```python
from build123d import *

# Parameters (mm, degrees)
F1_DEPTH = 2
F3_DEPTH = 2
F5_DEPTH = 2
F6_R     = 1


with BuildPart() as f1:
    # F0 (on Top) → F1 (new body)
    with BuildSketch(Plane.XY):
        Polygon((-13.435029, 6.363961), (-2.071068, -5), (14, -5), (14, 4), (1.656854, 4), (-7.071068, 12.727922), align=None)
    extrude(amount=F1_DEPTH)

    # F2 (on face) → F3 (join)
    with BuildSketch(Plane.XY.offset(2)):
        Polygon((-12.020815, 7.778175), (-13.435029, 6.363961), (-2.071068, -5), (14, -5), (14, -3), (-1.242641, -3), align=None)
    extrude(amount=F3_DEPTH)

    # F4 (on face) → F5 (join)
    with BuildSketch(Plane.XY.offset(4)):
        Polygon((-7.071068, 12.727922), (-12.020815, 7.778175), (-13.435029, 6.363961), (-2.071068, -5), (14, -5), (14, -3), (14, 4), (1.656854, 4), align=None)
    extrude(amount=F5_DEPTH)

    # F6
    f6_edges = [f1.edges().sort_by_distance(p)[0] for p in [
        (-13.435029, 6.363961, 3),
        (-7.753048, 0.681981, 6),
        (-2.071068, -5, 3),
        (-7.753048, 0.681981, 0),
        (5.964466, -5, 6),
        (14, -5, 3),
        (5.964466, -5, 0),
        (-10.253048, 9.545942, 0),
        (14, -0.5, 0),
        (7.828427, 4, 0),
        (-2.707107, 8.363961, 0),
        (14, -0.5, 6),
        (7.828427, 4, 6),
        (-2.707107, 8.363961, 6),
        (-10.253048, 9.545942, 6),
    ]]
    fillet(f6_edges, radius=F6_R)


solid = f1.part
```
Model file for the job. Use its own axes, mm. A direction names the side the tool comes from. Coordinates: 2 decimals unless noted, no trailing zeros. Loops run counter-clockwise (first coordinate to the right, second up) from the corner with the lowest first, then second, coordinate; pieces in that order, holes last. Notation, with made-up numbers: (36, -5.5) - (40, -5.5) arc R17 ccw to (40, 21.5) - close; hole circle Ø9 at (53, -28). An arc over 180 degrees is marked (long way). Answer as a JSON object with one key per item and string values. Group by question number.
(1) Tool access for faces 1 (the face through (5.774, -4.715, 5.699)), 2 (the face through (1, 3, 4)), 3 (the face through (7.532, 3.715, 5.699)): list every direction of +Z, -Z, +X, -X, +Y, -Y with a clear straight run to the whole face (end or side of a thin tool).
(2) Flat gauge pin, fed straight in: pin 1 (1.1 mm diameter, centred on x = 8, z = 1.5, fed in from +Y). Where does the tip first touch, or does it go through?
(3) Cut at A-A (x = 11.25). Give the cut face in (y, z), then the cut area to 3 significant figures.
(4) Probe line 1 along Z through (x, y) = (2, -1.75); line 2 along Y through (x, z) = (6.75, 1.75); line 3 along Z through (x, y) = (-10, 9.5). List the from-to ranges inside material, lowest first.
(5) Two-plate mould, pull along Z, no slides. Class faces 4 (the face through (13.715, 0.056, 5.699)), 5 (the face through (-6.556, 2.314, 2.986)), 6 (the face through (7.9, 4, 4.5)): released by +Z, released by -Z, zero draft, split by the parting line, or undercut.
(6) Cut at B-B (z = 2.5). Give the cut face in (x, y), then the cut area to 3 significant figures.
Geometry says:
{
 "1": {"face 1": "+Z, +X, -X, -Y", "face 2": "+X, +Y", "face 3": "+Z, +X, +Y"},
 "2": {"pin 1": "stops at y = 4"},
 "3": {"outline": "(-5, 1) arc R1 ccw to (-4, 0) - (3, 0) arc R1 ccw to (4, 1) - (4, 2) - (-3, 2) - (-3, 4) - (4, 4) - (4, 5) arc R1 ccw to (3, 6) - (-4, 6) arc R1 ccw to (-5, 5) - close", "area": "39.1 mm^2"},
 "4": {"line 1": "z = 0 to 2, 4 to 6", "line 2": "y = -5 to 4", "line 3": "z = 0.39 to 2, 4 to 5.61"},
 "5": {"face 4": "released by +Z", "face 5": "undercut", "face 6": "zero draft"},
 "6": {"outline": "(-12.73, 5.66) - (-2.36, -4.71) arc R1 ccw to (-1.66, -5) - (13, -5) arc R1 ccw to (14, -4) - (14, -3) - (-1.24, -3) - (-12.02, 7.78) - (-12.73, 7.07) arc R1 ccw to start", "area": "62.2 mm^2"}
}
